from build123d import *

# Parameters (mm, degrees)
EXTRUDE_1_DEPTH              = 30
SKETCH_3_R                   = 5
CUT_EXTRUDE_1_DEPTH          = 57.400354609
SKETCH_6_R                   = 3
CUT_EXTRUDE_3_DEPTH          = 57.400354609
SKETCH_9_W                   = 4
SKETCH_9_H                   = 9
EXTRUDE_3_DEPTH              = 3
SKETCH_10_W                  = 9
SKETCH_10_H                  = 28
CUT_EXTRUDE_4_DEPTH          = 1
HOLE_START                   = 1
HOLE_WIZARD_M3_1_OUTLINE_R   = 1.25
HOLE_WIZARD_M3_1_DEPTH       = 3
CUT_EXTRUDE_5_DEPTH          = 59.821764679
CHAMFER_1_SIZE               = 10
HOLE_START_2                 = 42
HOLE_WIZARD_M2_5_3_OUTLINE_R = 1.025
HOLE_WIZARD_M2_5_3_DEPTH     = 3
CUT_EXTRUDE_6_REACH          = 58.4
SKETCH_18_R                  = 6
FILLET_2_R                   = 2
FILLET_3_R                   = 2
HOLE_WIZARD_M2_1_D           = 1.6


# Read off the part's stored shape, not the designer's step: M3 螺纹孔1, M2.5 螺纹孔3
with BuildPart() as part:
    # 草图2 → 凸台-拉伸1 (new body)
    with BuildSketch(Plane.XY):
        Polygon((16, 42), (4, 42), (4, 0), (0, 0), (0, 45), (16, 45), align=None)
    extrude(amount=EXTRUDE_1_DEPTH)

    # 草图3 → 切除-拉伸1 (cut, through all)
    with BuildSketch(Plane(origin=(0, 0, 30), x_dir=(0, 0, -1), z_dir=(1, 0, 0))):
        with Locations(Location((15, 12.5, 0), (0, 0, 270))):
            Circle(SKETCH_3_R)
    extrude(amount=CUT_EXTRUDE_1_DEPTH, mode=Mode.SUBTRACT)

    # 草图6 → 切除-拉伸3 (cut, through all)
    with BuildSketch(Plane(origin=(0, 45, 0), x_dir=(1, 0, 0), z_dir=(0, 1, 0))):
        with Locations(Location((8, -23, 0), (0, 0, 270))):
            Circle(SKETCH_6_R)
        with Locations(Location((8, -7, 0), (0, 0, 270))):
            Circle(SKETCH_6_R)
    extrude(amount=-CUT_EXTRUDE_3_DEPTH, mode=Mode.SUBTRACT)

    # 草图9 → 凸台-拉伸3 (add)
    with BuildSketch(Plane(origin=(0, 45, 0), x_dir=(1, 0, 0), z_dir=(0, 1, 0))):
        with Locations((2, -15)):
            Rectangle(SKETCH_9_W, SKETCH_9_H)
    extrude(amount=EXTRUDE_3_DEPTH)

    # 草图10 → 切除-拉伸4 (cut)
    with BuildSketch(Plane.ZY):
        with Locations((15, 34)):
            Rectangle(SKETCH_10_W, SKETCH_10_H)
    extrude(amount=-CUT_EXTRUDE_4_DEPTH, mode=Mode.SUBTRACT)

    # M3 螺纹孔1 outline → M3 螺纹孔1 (cut)
    with BuildSketch(Plane.YZ.offset(HOLE_START)):
        with Locations((25, 15)):
            Circle(HOLE_WIZARD_M3_1_OUTLINE_R)
        with Locations((45, 15)):
            Circle(HOLE_WIZARD_M3_1_OUTLINE_R)
    extrude(amount=HOLE_WIZARD_M3_1_DEPTH, mode=Mode.SUBTRACT)

    # 草图13 → 切除-拉伸5 (cut, through all)
    with BuildSketch(Plane.ZY):
        with BuildLine():
            Line((27, 37.5), (27, 22.5))
            ThreePointArc((27, 22.5), (25, 20.5), (23, 22.5))
            Line((23, 22.5), (23, 37.5))
            ThreePointArc((23, 37.5), (25, 39.5), (27, 37.5))
        make_face()
        with BuildLine():
            Line((3, 37.5), (3, 22.5))
            ThreePointArc((3, 22.5), (5, 20.5), (7, 22.5))
            Line((7, 22.5), (7, 37.5))
            ThreePointArc((7, 37.5), (5, 39.5), (3, 37.5))
        make_face()
    extrude(amount=-CUT_EXTRUDE_5_DEPTH, mode=Mode.SUBTRACT)

    # 倒角1
    chamfer_1_edges = [part.edges().sort_by_distance(p)[0] for p in [
        (2, 0, 30),
        (2, 0, 0),
    ]]
    chamfer(chamfer_1_edges, length=CHAMFER_1_SIZE)

    # M2.5 螺纹孔3 outline → M2.5 螺纹孔3 (cut)
    with BuildSketch(Plane(origin=(0, 0, 0), x_dir=(1, 0, 0), z_dir=(0, 1, 0)).offset(HOLE_START_2)):
        with Locations((3, -27)):
            Circle(HOLE_WIZARD_M2_5_3_OUTLINE_R)
        with Locations((13, -27)):
            Circle(HOLE_WIZARD_M2_5_3_OUTLINE_R)
        with Locations((13, -3)):
            Circle(HOLE_WIZARD_M2_5_3_OUTLINE_R)
        with Locations((3, -3)):
            Circle(HOLE_WIZARD_M2_5_3_OUTLINE_R)
    extrude(amount=HOLE_WIZARD_M2_5_3_DEPTH, mode=Mode.SUBTRACT)

    # 草图18 → 切除-拉伸6 (cut, up to next)
    with BuildSketch(Plane(origin=(0, 45, 0), x_dir=(1, 0, 0), z_dir=(0, 1, 0)), mode=Mode.PRIVATE) as cut_extrude_6_sk1:
        with Locations((18, -15)):
            Circle(SKETCH_18_R)
    cut_extrude_6_tool1 = extrude(cut_extrude_6_sk1.sketch, amount=-CUT_EXTRUDE_6_REACH, mode=Mode.PRIVATE) & part.part
    add(cut_extrude_6_tool1.solids().sort_by_distance((18, 45, 15))[0], mode=Mode.SUBTRACT)

    # 圆角2
    fillet_2_edges = [part.edges().sort_by_distance(p)[0] for p in [
        (16, 43.5, 30),
        (16, 43.5, 20.656854249),
        (16, 43.5, 9.343145751),
        (16, 43.5, 0),
    ]]
    fillet(fillet_2_edges, radius=FILLET_2_R)

    # 圆角3
    fillet_3_edges = [part.edges().sort_by_distance(p)[0] for p in [
        (0.5, 20, 10.5),
        (0.5, 20, 19.5),
    ]]
    fillet(fillet_3_edges, radius=FILLET_3_R)

    # M2 螺纹孔1 (through all)
    with Locations(Plane(origin=(4, 17.75, 24.09326674), x_dir=(0, 1, 0), z_dir=(1, 0, 0))):
        with Locations((0, 0), (0, -18.18653348), (-15.75, -9.09326674)):
            Hole(HOLE_WIZARD_M2_1_D / 2)


solid = part.part
Source: CAD feature listing. Evaluate the final solid. Frame: model axes, mm. A direction names the side the tool comes from. Round coordinates to 2 decimals unless told otherwise and drop trailing zeros. Loops run counter-clockwise (first coordinate to the right, second up) from the corner with the lowest first, then second, coordinate; pieces in that order, holes last. Notation, with made-up numbers: M 20,-14.5 L 29,-14.5 A38 cw 29,24.5 Z; hole C 62.5,6 d9. An arc over 180 degrees is marked long. Answer as CSV lines item,"result".
Q1. Cut plane D-D (y = 28). Return the cut outline in (x, z), plus the area to 3 significant figures.
Verdict:
outline,"M 0,0 L 4,0 L 4,3 L 0,3 Z; M 0,7 L 4,7 L 4,23 L 0,23 L 0,19.5 L 1,19.5 L 1,10.5 L 0,10.5 Z; M 0,27 L 4,27 L 4,30 L 0,30 Z"
area,"79.0 mm^2"
Q2. Cut plane B-B (z = 15). Return the cut outline in (x, y), plus the area to 3 significant figures.
Verdict:
outline,"M 0,0 L 4,0 L 4,1.2 L 0,1.2 Z; M 0,2.8 L 4,2.8 L 4,7.5 L 0,7.5 Z; M 0,17.5 L 4,17.5 L 4,23.75 L 1,23.75 L 1,20 L 0,20 Z; M 1,26.25 L 4,26.25 L 4,42 L 12,42 L 12,45 L 4,45 L 4,43.75 L 1,43.75 Z; M 1,46.25 L 4,46.25 L 4,48 L 1,48 Z"
area,"127 mm^2"
Q3. Reachability of faces 4 (the face through (2, 20.5, 25)), 5 (the face through (15.74, 43.52, 9.06)), 6 (the face through (10, 42, 15)) from +Z, -Z, +X, -X, +Y, -Y: full face, straight path, thin tool, end or side. Return the list, or none.
Verdict:
face 4,"+X, -X"
face 5,"+X, +Y, -Y"
face 6,"+Z, -Z, +X, -Y"
Q4. Cut plane C-C (y = 2). Return the cut outline in (x, z).
Verdict:
outline,"M 0,8 L 4,8 L 4,14.2 L 0,14.2 Z; M 0,15.8 L 4,15.8 L 4,22 L 0,22 Z"
Q5. Contact query for flat-ended pins moving along their axis: pin 1 (2 mm diameter, centred on x = 6.5, z = 16, fed in from +Y); pin 2 (1.3 mm diameter, centred on y = 17.75, z = 5.91, fed in from -X); pin 3 (1 mm diameter, centred on x = 3, z = 3, fed in from +Y); pin 4 (4 mm diameter, centred on y = 45, z = 15, fed in from -X). Output: stop coordinate, or through.
Verdict:
pin 1,"stops at y = 45"
pin 2,"passes through"
pin 3,"stops at y = 42"
pin 4,"stops at x = 1"
Q6. Pull-direction query (Y, two-part tool) for faces 1 (the face through (1.972, 17.381, 5.197)), 2 (the face through (4, 21, 15)), 3 (the face through (0.5, 20, 15)); classes: +Y half, -Y half, draft (parallel to the pull), parting line (faces both ways), or undercut.
Verdict:
face 1,"undercut"
face 2,"draft"
face 3,"+Y half"
Q7. Line query: line 1 along Z through (x, y) = (3, 42.9) (3 decimals); line 2 along Z through (x, y) = (3, 35); line 3 along X through (y, z) = (42.7, 3) (3 decimals). Output: solid intervals per line, ascending.
Verdict:
line 1,"z = 0 to 1.975, 4.025 to 25.975, 28.025 to 30"
line 2,"z = 0 to 3, 7 to 23, 27 to 30"
line 3,"x = 0 to 1.975, 4.025 to 11.975, 14.025 to 16"
Q8. Cut plane A-A (x = 8). Return the cut outline in (y, z).
Verdict:
outline,"M 42,0 L 45,0 L 45,4 L 42,4 Z; M 42,10 L 45,10 L 45,20 L 42,20 Z; M 42,26 L 45,26 L 45,30 L 42,30 Z"
